Here's how the part is built. I have some questions about the finished solid (model axes, mm). Round coordinates to 2 decimals unless told otherwise and drop trailing zeros. Write each loop counter-clockwise with the first axis right and the second up, starting at its lowest first coordinate (ties: lowest second). Pieces come first, ordered by that corner, then holes. Notation, with made-up numbers: (15, -31.5) - (35, -31.5) arc R13 ccw to (35, -24.5) - close; hole circle Ø9 at (61, 35.25). An arc over 180 degrees is marked (long way). Write item = value, one per line. Start each with the question number.
Item 1: For P1, Ø1.8, axis at y = 4.76, z = -31.75, coming from the -X side, with a flat end and sliding along its axis, tell me the tip position at first contact or that it passes through.
Item 2: If we section it at A-A (z = -31.75): Please give me the cut outline in (x, y) (1 decimal), and give its area (3 significant figures).
Item 3: If I drill on line 1 along Y through (x, z) = (5, -31.75) (3 decimals); line 2 along Z through (x, y) = (-3, 9); line 3 along X through (y, z) = (8.75, -25.5), over which ranges is the centre line in solid material (lowest first)? Write a range as [from, to].
Item 4: If we section it at B-B (y = 4): Please give me the cut outline in (x, z).
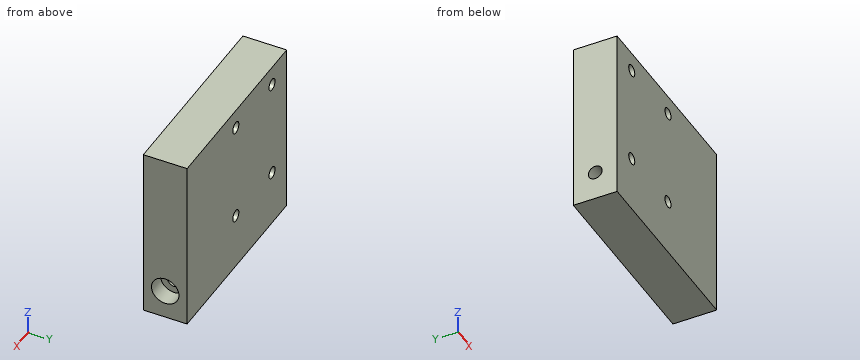
Autodesk Inventor part; units mm, degrees
ref_plane "YZ Plane" through (0, 0, 0) normal (1, 0, 0) x (0, 1, 0)
ref_plane "XZ Plane" through (0, 0, 0) normal (0, 1, 0) x (-1, 0, 0)
ref_plane "XY Plane" through (0, 0, 0) normal (0, 0, 1) x (1, 0, 0)
sketch "Sketch1" plane through (0, 0, 0) normal (0, 1, 0) x (-1, 0, 0)
  line L0 (-16.3555, 0) -> (25.5545, 0)
  line L1 (25.5545, 0) -> (25.5545, -38.1)
  line L2 (25.5545, -38.1) -> (-16.3555, -38.1)
  line L3 (-16.3555, -38.1) -> (-16.3555, 0)
  point P0 (0, 0)
  dimension "d0" = 41.91
  dimension "d1" = 38.1
extrude "Extrusion1" add sketch "Sketch1" along normal blind 9.525
sketch "Sketch2" plane through (16.3555, 0, 0) normal (1, 0, 0) x (0, 0, -1)
  circle A0 centre (31.75, 4.7625) radius 1.4986
  line L0 (0, 0) -> (38.1, 0)
  line L1 (38.1, 0) -> (38.1, 9.525)
  dimension "d4" = 2.9972
  dimension "d5" = 4.7625
  dimension "d6" = 6.35
extrude "Extrusion2" cut sketch "Sketch2" against normal through all
sketch "Sketch3" plane through (16.3555, 0, 0) normal (1, 0, 0) x (0, 0, -1)
  circle A0 centre (31.75, 4.7625) radius 1.4986
  circle A1 centre (31.75, 4.7625) radius 2.9845
  circle A2 centre (31.75, 4.7625) radius 1.4986
  point P0 (0, 0)
  dimension "d9" = 5.969
extrude "Extrusion3" cut sketch "Sketch3" against normal blind 3.81
sketch "Sketch4" plane through (0, 9.525, 0) normal (0, 1, 0) x (1, 0, 0)
  line L0 (-19.3894, 4.2047) -> (-4.1494, 4.2047)
  line L1 (-4.1494, 4.2047) -> (-4.1494, 25.7947)
  line L2 (-4.1494, 25.7947) -> (-19.3894, 25.7947)
  line L3 (-19.3894, 25.7947) -> (-19.3894, 4.2047)
  line L4 (16.3555, 38.1) -> (-25.5545, 38.1)
  line L5 (-25.5545, 38.1) -> (-25.5545, 0)
  circle A0 centre (-19.3894, 4.2047) radius 1.27
  circle A1 centre (-4.1494, 4.2047) radius 1.27
  circle A2 centre (-4.1494, 25.7947) radius 1.27
  circle A3 centre (-19.3894, 25.7947) radius 1.27
  point P0 (0, 0)
  point P1 (-19.3894, 14.9997)
  dimension "d12" = 21.59
  dimension "d14" = 15.24
  dimension "d16" = 2.54
  dimension "d17" = 2.54
  dimension "d20" = 2.54
extrude "Extrusion4" cut sketch "Sketch4" against normal through all contours L3 A0 L0 | L0 A0 L3 | A1 L1 L0 | L0 L1 A1 | A3 L2 L3 | L3 L2 A3 | A2 L2 L1 | L1 L2 A2
properties part number "sensor bendor"
Reply:
q1.P1 = through
q2.outline = (-25.6, 0) - (16.4, 0) - (16.4, 1.8) - (12.5, 1.8) - (12.5, 3.3) - (-25.6, 3.3) - close; (-25.6, 6.3) - (12.5, 6.3) - (12.5, 7.7) - (16.4, 7.7) - (16.4, 9.5) - (-25.6, 9.5) - close
q2.area = 262 mm2
q3.line_1 = [0, 3.264], [6.261, 9.525]
q3.line_2 = [-38.1, -26.33], [-25.25, -4.74], [-3.66, 0]
q3.line_3 = [-25.55, -20.62], [-18.15, -5.38], [-2.91, 16.36]
q4.outline = (-25.55, -38.1) - (16.36, -38.1) - (16.36, -34.64) - (12.55, -34.64) - (12.55, -33.04) - (-25.55, -33.04) - close; (-25.55, -30.46) - (12.55, -30.46) - (12.55, -28.86) - (16.36, -28.86) - (16.36, 0) - (-25.55, 0) - close; hole circle Ø2.54 at (-19.39, -25.79); hole circle Ø2.54 at (-19.39, -4.2); hole circle Ø2.54 at (-4.15, -25.79); hole circle Ø2.54 at (-4.15, -4.2)
